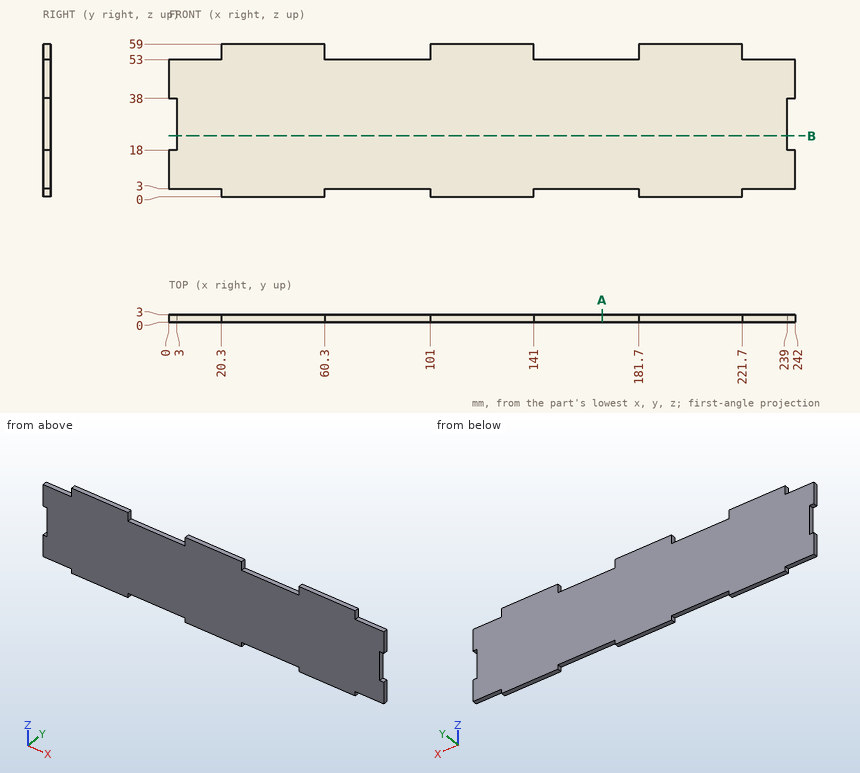
Geometry: see drawing. Coordinates: mm, zero at the bounding-box minimum. Round coordinates to 2 decimals unless told otherwise and drop trailing zeros. Loops run counter-clockwise (first coordinate to the right, second up) from the corner with the lowest first, then second, coordinate; pieces in that order, holes last. Notation, with made-up numbers: (24.25, 24) -> (45.25, 24) arc R22 ccw to (45.25, 34) -> close; hole circle Ø9 at (-33.5, -14). An arc over 180 degrees is marked (long way). Use one line per item in the form item = value. Start each with the question number.
Item 1: Contact query for flat-ended pins moving along their axis: pin 1 Ø1 at (x, y) = (166, 0.5) entering from -Z; pin 2 Ø1.5 at (x, y) = (236.5, 1.5) entering from +Z; pin 3 Ø0.9 at (y, z) = (2, 2) entering from -X. Output: stop coordinate, or through.
Item 2: Section query B-B on z = 23.5. Return the cut outline in (x, y), then the cut area to 3 significant figures.
Item 3: Section query A-A on x = 167.5. Return the cut outline in (y, z), then the cut area to 3 significant figures.
Item 4: Material intervals for L1, parallel to X at y = 0.55, z = 54.5; L2, parallel to Z at x = 226.5, y = 1.8; L3, parallel to X at y = 1.9, z = 26, sorted ascending. Write a range as from..to.
Ans:
q1.pin_1 = 3
q1.pin_2 = 53
q1.pin_3 = 20.3
q2.outline = (3, 0) -> (239, 0) -> (239, 3) -> (3, 3) -> close
q2.area = 708 mm^2
q3.outline = (0, 3) -> (3, 3) -> (3, 53) -> (0, 53) -> close
q3.area = 150 mm^2
q4.L1 = 20.3..60.3, 101..141, 181.7..221.7
q4.L2 = 3..53
q4.L3 = 3..239
